Work out the finished part from the listing and answer in its coordinate system (mm). Round coordinates to 2 decimals unless told otherwise and drop trailing zeros. Order: outer loops, then holes, each group sorted by start corner. A loop starts at its lowest first (then second) coordinate and runs counter-clockwise, first axis right, second up. Notation, with made-up numbers: (-28.75, 1.25) - (-10.75, 1.25) arc R33 ccw to (-10.75, 35.25) - close; hole circle Ø3 at (41, 28.25). An arc over 180 degrees is marked (long way). Put each result on its own line as item: value.
```python
from build123d import *

# Parameters (mm, degrees)
BOSS_EXTRUDE1_DEPTH              = 11.1125
F_97_0_0059_DIAMETER_HOLE1_D     = 2.9464
F_97_0_0059_DIAMETER_HOLE1_DEPTH = 25.4
F_97_0_0059_DIAMETER_HOLE1_TIP   = 0.885187864


with BuildPart() as part:
    # Sketch1 → Boss-Extrude1 (new body)
    with BuildSketch(Plane(origin=(0, 0, 0), x_dir=(1, 0, 0), z_dir=(0, 1, 0))):
        Polygon((2.749630657, 0), (1.374815329, 2.38125), (-1.374815329, 2.38125), (-2.749630657, 0), (-1.374815329, -2.38125), (1.374815329, -2.38125), align=None)
    extrude(amount=BOSS_EXTRUDE1_DEPTH)

    # #97 (0.0059) Diameter Hole1
    with Locations(Plane(origin=(0, 11.1125, 0), x_dir=(1, 0, 0), z_dir=(0, 1, 0))):
        with Locations((0, 0)):
            Hole(F_97_0_0059_DIAMETER_HOLE1_D / 2, depth=F_97_0_0059_DIAMETER_HOLE1_DEPTH)
            with Locations((0, 0, -(F_97_0_0059_DIAMETER_HOLE1_DEPTH + F_97_0_0059_DIAMETER_HOLE1_TIP / 2))):  # 118° drill point
                Cone(0, F_97_0_0059_DIAMETER_HOLE1_D / 2, F_97_0_0059_DIAMETER_HOLE1_TIP, mode=Mode.SUBTRACT)


solid = part.part
```
1) Straight lines are drawn through the part: L1, parallel to Z at x = 0, y = 2.5; L2, parallel to X at y = 6.75, z = 0.3; L3, parallel to X at y = 6, z = -1.15. For each, find the intervals that lie inside material, in ascending order. Write a range as from..to.
Findings below:
L1: z = -2.38..-1.47, 1.47..2.38
L2: x = -2.58..-1.44, 1.44..2.58
L3: x = -2.09..-0.92, 0.92..2.09
2) Given pin 1 Ø1.5 at (y, z) = (8, 0.5) entering from +X, flat-ended and moving along its own axis, determine where the tip first touches the part or whether it passes through.
Findings below:
pin 1: stops at x = 2.75
3) A cutting plane is placed at A-A on x = 0. Write down the section's boundary in (y, z), then the cut area to 3 significant figures.
Findings below:
outline: (0, -2.38) - (11.11, -2.38) - (11.11, -1.47) - (0, -1.47) - close; (0, 1.47) - (11.11, 1.47) - (11.11, 2.38) - (0, 2.38) - close
area: 20.2 mm2
4) A cutting plane is placed at B-B on z = 0.95. Write down the section's boundary in (x, y), then the cut area to 3 significant figures.
Findings below:
outline: (-2.2, 0) - (-1.13, 0) - (-1.13, 11.11) - (-2.2, 11.11) - close; (1.13, 0) - (2.2, 0) - (2.2, 11.11) - (1.13, 11.11) - close
area: 23.9 mm2
5) For a pull along Z with two mould halves and no side action, classify faces 1 (the flat face through (1.2, 0, -1.1)), 2 (the cylindrical face through (-1.405, 5.478, -0.443)), 3 (the flat face through (0, 5, -2.381)), 4 (the flat face through (-2.072, 5.478, 1.174)) as pulls with the +Z half, pulls with the -Z half, needs draft (parallel to the pull), parting line crosses it, or undercut.
Findings below:
face 1: needs draft
face 2: undercut
face 3: pulls with the -Z half
face 4: pulls with the +Z half
6) A cutting plane is placed at D-D on z = -1.85. Write down the section's boundary in (x, y).
Findings below:
outline: (-1.68, 0) - (1.68, 0) - (1.68, 11.11) - (-1.68, 11.11) - close
7) A cutting plane is placed at C-C on y = 10.5. Write down the section's boundary in (x, z).
Findings below:
outline: (-2.75, 0) - (-1.37, -2.38) - (1.37, -2.38) - (2.75, 0) - (1.37, 2.38) - (-1.37, 2.38) - close; hole circle Ø2.95 at (0, 0)
